from build123d import *

# Parameters (mm, degrees)
SKETCH_W   = 90
SKETCH_H   = 60
SKETCH_R   = 2.25
SKETCH_R_2 = 2
SKETCH_R_3 = 1.5
SKETCH_W_2 = 7
SKETCH_H_2 = 4
SKETCH_W_3 = 19
SKETCH_H_3 = 18
PAD_DEPTH  = 3


with BuildPart() as part:
    # Sketch → Pad (new body)
    with BuildSketch(Plane.XY):
        with Locations((45, 30)):
            Rectangle(SKETCH_W, SKETCH_H)
        with Locations((10, 5)):
            Circle(SKETCH_R, mode=Mode.SUBTRACT)
        with Locations((33, 24)):
            Circle(SKETCH_R_2, mode=Mode.SUBTRACT)
        with Locations((33, 36)):
            Circle(SKETCH_R_2, mode=Mode.SUBTRACT)
        with Locations((33, 30)):
            Circle(SKETCH_R_2, mode=Mode.SUBTRACT)
        with Locations((10, 55)):
            Circle(SKETCH_R, mode=Mode.SUBTRACT)
        with Locations((14, 11)):
            Circle(SKETCH_R_3, mode=Mode.SUBTRACT)
        with Locations((5, 11)):
            Circle(SKETCH_R_3, mode=Mode.SUBTRACT)
        with Locations((14, 49)):
            Circle(SKETCH_R_3, mode=Mode.SUBTRACT)
        with Locations((5, 49)):
            Circle(SKETCH_R_3, mode=Mode.SUBTRACT)
        with Locations((10, 16)):
            Rectangle(SKETCH_W_2, SKETCH_H_2, mode=Mode.SUBTRACT)
        with Locations((10, 44)):
            Rectangle(SKETCH_W_2, SKETCH_H_2, mode=Mode.SUBTRACT)
        with Locations((10.5, 30)):
            Rectangle(SKETCH_W_3, SKETCH_H_3, mode=Mode.SUBTRACT)
    pad = extrude(amount=PAD_DEPTH)

    # Mirrored: Pad across face of Pad
    add(pad.mirror(Plane(origin=(90, 30, 1.5), x_dir=(0, 1, 0), z_dir=(1, 0, 0))))


solid = part.part
The model under review builds one solid part; all positions refer to its coordinate system, in mm. Round coordinates to 2 decimals unless told otherwise and drop trailing zeros. Loops run counter-clockwise (first coordinate to the right, second up) from the corner with the lowest first, then second, coordinate; pieces in that order, holes last. Notation, with made-up numbers: (4.25, 17.25) -> (61.25, 17.25) arc R19 cw to (61.25, 43.25) -> close; hole circle Ø4 at (-36.5, 78). An arc over 180 degrees is marked (long way). Return JSON: item names as keys, results as strings.
(1) Add section B-B on x = 170. Write out the cut boundary in (y, z).
Solved:
{"outline": "(0, 0) -> (2.75, 0) -> (2.75, 3) -> (0, 3) -> close; (7.25, 0) -> (14, 0) -> (14, 3) -> (7.25, 3) -> close; (18, 0) -> (21, 0) -> (21, 3) -> (18, 3) -> close; (39, 0) -> (42, 0) -> (42, 3) -> (39, 3) -> close; (46, 0) -> (52.75, 0) -> (52.75, 3) -> (46, 3) -> close; (57.25, 0) -> (60, 0) -> (60, 3) -> (57.25, 3) -> close"}
(2) Add section C-C on x = 147. Write out the cut boundary in (y, z), plus the area to 3 significant figures.
Solved:
{"outline": "(0, 0) -> (22, 0) -> (22, 3) -> (0, 3) -> close; (26, 0) -> (28, 0) -> (28, 3) -> (26, 3) -> close; (32, 0) -> (34, 0) -> (34, 3) -> (32, 3) -> close; (38, 0) -> (60, 0) -> (60, 3) -> (38, 3) -> close", "area": "144 mm2"}
(3) The part is to be moulded in two halves that separate along Y. For faces 1 (the flat face through (166.5, 16, 1)), 2 (the flat face through (170, 18, 1)), say which applies: released by +Y, released by -Y, zero draft, split by the parting line, or undercut.
Solved:
{"face 1": "undercut", "face 2": "undercut"}
(4) For line 1 (X direction, y = 42.5, z = 0.3); line 2 (X direction, y = 32.5, z = 0.55); line 3 (Y direction, x = 14, z = 1.5), list the stretches that pass through material, from the lowest coordinate up.
Solved:
{"line 1": "0 to 6.5, 13.5 to 166.5, 173.5 to 180", "line 2": "0 to 1, 20 to 160, 179 to 180", "line 3": "0 to 9.5, 12.5 to 21, 39 to 47.5, 50.5 to 60"}
(5) For pin 1 (2.5 mm diameter, centred on x = 5, y = 11, fed in from +Z); pin 2 (8 mm diameter, centred on x = 123.5, y = 6.5, fed in from -Z), all flat-tipped, find the tip position at first contact; note any pin that passes through.
Solved:
{"pin 1": "through", "pin 2": "z = 0"}
(6) Add section A-A on y = 55. Write out the cut boundary in (x, z).
Solved:
{"outline": "(0, 0) -> (7.75, 0) -> (7.75, 3) -> (0, 3) -> close; (12.25, 0) -> (167.75, 0) -> (167.75, 3) -> (12.25, 3) -> close; (172.25, 0) -> (180, 0) -> (180, 3) -> (172.25, 3) -> close"}
(7) Add section D-D on y = 36. Write out the cut boundary in (x, z).
Solved:
{"outline": "(0, 0) -> (1, 0) -> (1, 3) -> (0, 3) -> close; (20, 0) -> (31, 0) -> (31, 3) -> (20, 3) -> close; (35, 0) -> (145, 0) -> (145, 3) -> (35, 3) -> close; (149, 0) -> (160, 0) -> (160, 3) -> (149, 3) -> close; (179, 0) -> (180, 0) -> (180, 3) -> (179, 3) -> close"}
